Can you work these out from the model? Positions are in its coordinate system, mm. A direction names the side the tool comes from. Give positions to 0.01 mm unless a question says otherwise; leave off trailing zeros. Loops run counter-clockwise (first coordinate to the right, second up) from the corner with the lowest first, then second, coordinate; pieces in that order, holes last. Notation, with made-up numbers: (-34, -9) -> (-18, -9) arc R23 ccw to (-18, 2) -> close; hole circle Ø4 at (55, 17.25). An arc over 180 degrees is marked (long way). Return JSON: item names as keys, results as strings. Group by question number.
Q1. Suppose I cut it at B-B, the plane x = 12.5. Please give me the cut outline in (y, z), and give its area (3 significant figures).
Q2. Suppose I cut it at A-A, the plane y = -12. Please give me the cut outline in (x, z), and give its area (3 significant figures).
Q3. I need wall thicknesses on line 1 along Z through (x, y) = (-11, -9); line 2 along X through (y, z) = (0.5, 132); line 3 along Z through (x, y) = (-45, 20). Which ranges of each line are inside material? Lowest first, please. Write a range as [from, to].
Q4. Will these pins go through, and if not, where does the flat tip stop? pin 1 (5 mm diameter, centred on x = 39.5, y = 1.5, fed in from +Z); pin 2 (10 mm diameter, centred on y = -7.5, z = 87, fed in from +X); pin 3 (2 mm diameter, centred on x = -7, z = 53.5, fed in from -Y).
Q5. Which directions (+Z, -Z, +X, -X, +Y, -Y) give clear straight access to the entire face, cutting with the end or side of a thin tool? Please do faces 1 (the flat face through (0, 8.2, 2.5)), 2 (the flat face through (-1, 25, -25)), 3 (the cylindrical face through (5.36, 8.41, 154.96)).
Q6. Suppose I cut it at C-C, the plane x = 0. Please give me the cut outline in (y, z), and give its area (3 significant figures).
Q7. Suppose I cut it at D-D, the plane z = 118.5. Please give me the cut outline in (x, y).
```python
from build123d import *

# Parameters (mm, degrees)
F0_R     = 10.017948
F1_DEPTH = 2.5
F2_R     = 8.037712
F3_DEPTH = 150
F4_R     = 9.974269
F6_DEPTH = 5
F5_W     = 100
F5_H     = 50
F7_DEPTH = 50
F8_SIZE  = 5.08


with BuildPart() as f1:
    # F0 (on Top) → F1 (new body)
    with BuildSketch(Plane.XY):
        Circle(F0_R)
    extrude(amount=F1_DEPTH)

    # F2 (on face) → F3 (join)
    with BuildSketch(Plane.XY.offset(2.5)):
        Circle(F2_R)
    extrude(amount=F3_DEPTH)

    # F4 (on face) → F6 (join)
    with BuildSketch(Plane.XY.offset(152.5)):
        Circle(F4_R)
    extrude(amount=F6_DEPTH)

    # F5 (on Top) → F7 (join)
    with BuildSketch(Plane.XY):
        Rectangle(F5_W, F5_H)
    extrude(amount=-F7_DEPTH)

    # F8
    f8_edges = [f1.edges().sort_by_distance(p)[0] for p in [
        (-50, -25, -25),
        (50, -25, -25),
        (0, -25, 0),
        (0, -25, -50),
        (50, 25, -25),
        (-50, 25, -25),
        (0, 25, 0),
        (0, 25, -50),
        (-50, 0, -50),
        (50, 0, -50),
        (50, 0, 0),
        (-50, 0, 0),
    ]]
    chamfer(f8_edges, length=F8_SIZE)


solid = f1.part
```
Ans:
{
 "1": {"outline": "(-25, -44.92) -> (-19.92, -50) -> (19.92, -50) -> (25, -44.92) -> (25, -5.08) -> (19.92, 0) -> (-19.92, 0) -> (-25, -5.08) -> close", "area": "2,450 mm^2"},
 "2": {"outline": "(-50, -44.92) -> (-44.92, -50) -> (44.92, -50) -> (50, -44.92) -> (50, -5.08) -> (44.92, 0) -> (-44.92, 0) -> (-50, -5.08) -> close", "area": "4,950 mm^2"},
 "3": {"line 1": "z = [-50, 0]", "line 2": "x = [-8.02, 8.02]", "line 3": "z = [-49.84, -0.16]"},
 "4": {"pin 1": "stops at z = 0", "pin 2": "stops at x = 7.64", "pin 3": "stops at y = -5.35"},
 "5": {"face 1": "none", "face 2": "+Z, -Z, +X, -X, +Y", "face 3": "+Z"},
 "6": {"outline": "(-25, -44.92) -> (-19.92, -50) -> (19.92, -50) -> (25, -44.92) -> (25, -5.08) -> (19.92, 0) -> (10.02, 0) -> (10.02, 2.5) -> (8.04, 2.5) -> (8.04, 152.5) -> (9.97, 152.5) -> (9.97, 157.5) -> (-9.97, 157.5) -> (-9.97, 152.5) -> (-8.04, 152.5) -> (-8.04, 2.5) -> (-10.02, 2.5) -> (-10.02, 0) -> (-19.92, 0) -> (-25, -5.08) -> close", "area": "5,010 mm^2"},
 "7": {"outline": "circle Ø16.08 at (0, 0)"}
}
